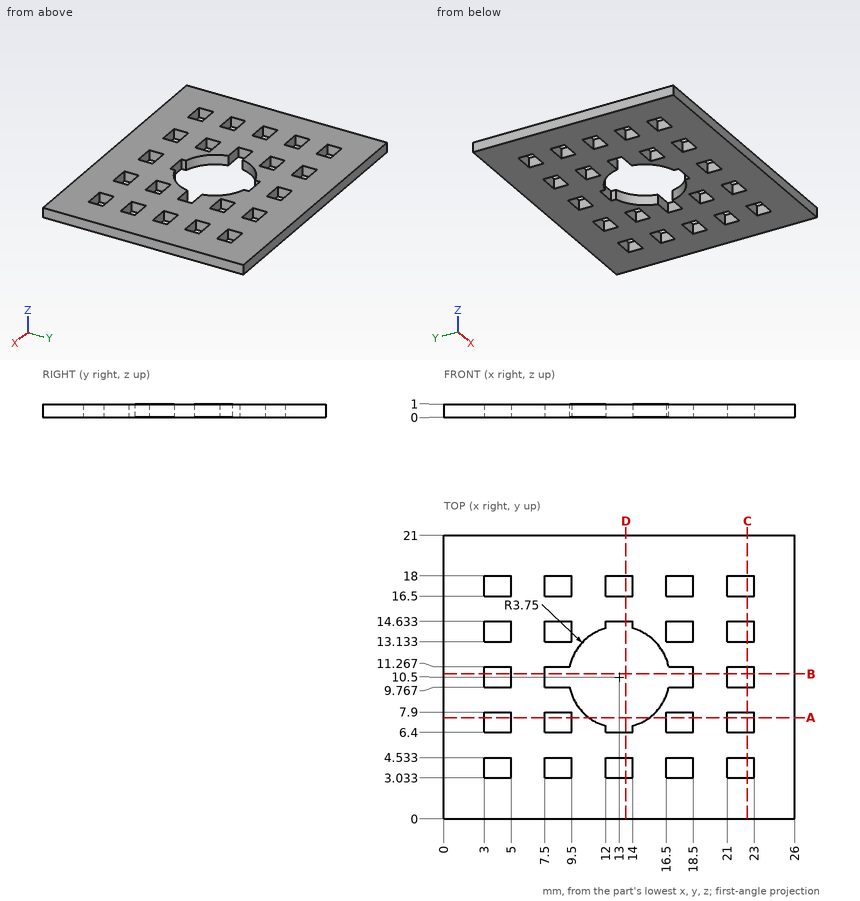
The drawing under review shows one solid part. Ordinate dimensions are in mm from its lowest x, y, z. Give positions to 0.01 mm unless a question says otherwise; leave off trailing zeros. Order: outer loops, then holes, each group sorted by start corner. A loop starts at its lowest first (then second) coordinate and runs counter-clockwise, first axis right, second up. Notation, with made-up numbers: (3.25, -26.5) - (19.25, -26.5) arc R21 ccw to (19.25, -7.5) - close; hole circle Ø5 at (10.5, 86). An arc over 180 degrees is marked (long way). Answer as a JSON object with one key per item and string values. Group by question number.
Item 1: Clearance check with a flat-ended pin moving along its axis: pin 1 Ø0.5 at (x, z) = (17.5, 0.5) entering from -Y. State where the tip first meets the part, or that it passes through.
Item 2: Take a section at C-C on x = 22.5. Give the boundary of the cut face in (y, z), and give its area (3 significant figures).
Item 3: Take a section at A-A on y = 7.5. Give the boundary of the cut face in (x, z).
Item 4: Take a section at B-B on y = 10.75. Give the boundary of the cut face in (x, z).
Item 5: Take a section at D-D on x = 13.5. Give the boundary of the cut face in (y, z).
Item 6: Wall thickness on line 1 along Y through (x, z) = (13.75, 0.55); line 2 along X through (y, z) = (11, 0.1); line 3 along Y through (x, z) = (9, 0.65): over which ranges is each line inside the solid? List them lowest first.
Reported:
{
 "1": {"pin 1": "y = 0"},
 "2": {"outline": "(0, 0) - (3.03, 0) - (3.03, 1) - (0, 1) - close; (4.53, 0) - (6.4, 0) - (6.4, 1) - (4.53, 1) - close; (7.9, 0) - (9.77, 0) - (9.77, 1) - (7.9, 1) - close; (11.27, 0) - (13.13, 0) - (13.13, 1) - (11.27, 1) - close; (14.63, 0) - (16.5, 0) - (16.5, 1) - (14.63, 1) - close; (18, 0) - (21, 0) - (21, 1) - (18, 1) - close", "area": "13.5 mm^2"},
 "3": {"outline": "(0, 0) - (3, 0) - (3, 1) - (0, 1) - close; (5, 0) - (7.5, 0) - (7.5, 1) - (5, 1) - close; (9.5, 0) - (10.75, 0) - (10.75, 1) - (9.5, 1) - close; (15.25, 0) - (16.5, 0) - (16.5, 1) - (15.25, 1) - close; (18.5, 0) - (21, 0) - (21, 1) - (18.5, 1) - close; (23, 0) - (26, 0) - (26, 1) - (23, 1) - close"},
 "4": {"outline": "(0, 0) - (3, 0) - (3, 1) - (0, 1) - close; (5, 0) - (7.5, 0) - (7.5, 1) - (5, 1) - close; (18.5, 0) - (21, 0) - (21, 1) - (18.5, 1) - close; (23, 0) - (26, 0) - (26, 1) - (23, 1) - close"},
 "5": {"outline": "(0, 0) - (3.03, 0) - (3.03, 1) - (0, 1) - close; (4.53, 0) - (6.4, 0) - (6.4, 1) - (4.53, 1) - close; (14.63, 0) - (16.5, 0) - (16.5, 1) - (14.63, 1) - close; (18, 0) - (21, 0) - (21, 1) - (18, 1) - close"},
 "6": {"line 1": "0 to 3.03, 4.53 to 6.4, 14.63 to 16.5, 18 to 21", "line 2": "0 to 3, 5 to 7.5, 18.5 to 21, 23 to 26", "line 3": "0 to 3.03, 4.53 to 6.4, 7.9 to 9.77, 11.27 to 13.13, 14.63 to 16.5, 18 to 21"}
}
